```python
from build123d import *

# Parameters (mm, degrees)
SKETCH1_W           = 23
SKETCH1_H           = 12
BOSS_EXTRUDE1_DEPTH = 24
BOSS_EXTRUDE2_DEPTH = 4.5
SKETCH3_R           = 2.5
BOSS_EXTRUDE3_DEPTH = 3
SKETCH4_R           = 0.85
CUT_EXTRUDE1_DEPTH  = 5
BOSS_EXTRUDE4_START = -4
SKETCH5_W           = 4.5
SKETCH5_H           = 12
SKETCH5_R           = 1.125
BOSS_EXTRUDE4_DEPTH = 2.5


with BuildPart() as part:
    # Sketch1 → Boss-Extrude1 (new body)
    with BuildSketch(Plane(origin=(0, 0, 0), x_dir=(1, 0, 0), z_dir=(0, 1, 0))):
        Rectangle(SKETCH1_W, SKETCH1_H)
    extrude(amount=BOSS_EXTRUDE1_DEPTH)

    # Sketch2 → Boss-Extrude2 (add)
    with BuildSketch(Plane(origin=(0, 24, 0), x_dir=(1, 0, 0), z_dir=(0, 1, 0))):
        with BuildLine():
            ThreePointArc((0.303829175, 2.999968125), (-2.71, 0), (0.303829175, -2.999968125))
            ThreePointArc((0.303829175, -2.999968125), (11.5, 0), (0.303829175, 2.999968125))
        make_face()
    extrude(amount=BOSS_EXTRUDE2_DEPTH)

    # Sketch3 → Boss-Extrude3 (add)
    with BuildSketch(Plane(origin=(0, 28.5, 0), x_dir=(1, 0, 0), z_dir=(0, 1, 0))):
        with Locations(Location((5.5, 0, 0), (0, 0, 270))):
            Circle(SKETCH3_R)
    extrude(amount=BOSS_EXTRUDE3_DEPTH)

    # Sketch4 → Cut-Extrude1 (cut)
    with BuildSketch(Plane(origin=(0, 31.5, 0), x_dir=(1, 0, 0), z_dir=(0, 1, 0))):
        with Locations(Location((5.5, 0, 0), (0, 0, 270))):
            Circle(SKETCH4_R)
    extrude(amount=-CUT_EXTRUDE1_DEPTH, mode=Mode.SUBTRACT)

    # Sketch5 → Boss-Extrude4 (add)
    # profile 1 of 2: a face of its own
    with BuildSketch(Plane(origin=(0, 24, 0), x_dir=(1, 0, 0), z_dir=(0, 1, 0)).offset(BOSS_EXTRUDE4_START)):
        with Locations((-13.75, 0)):
            Rectangle(SKETCH5_W, SKETCH5_H)
        with Locations(Location((-13.75, 0, 0), (0, 0, 270))):
            Circle(SKETCH5_R, mode=Mode.SUBTRACT)
    # profile 2 of 2: a face of its own
    with BuildSketch(Plane(origin=(0, 24, 0), x_dir=(1, 0, 0), z_dir=(0, 1, 0)).offset(BOSS_EXTRUDE4_START)):
        with Locations((13.75, 0)):
            Rectangle(SKETCH5_W, SKETCH5_H)
        with Locations(Location((13.75, 0, 0), (0, 0, 90))):
            Circle(SKETCH5_R, mode=Mode.SUBTRACT)
    extrude(amount=-BOSS_EXTRUDE4_DEPTH)


solid = part.part
```
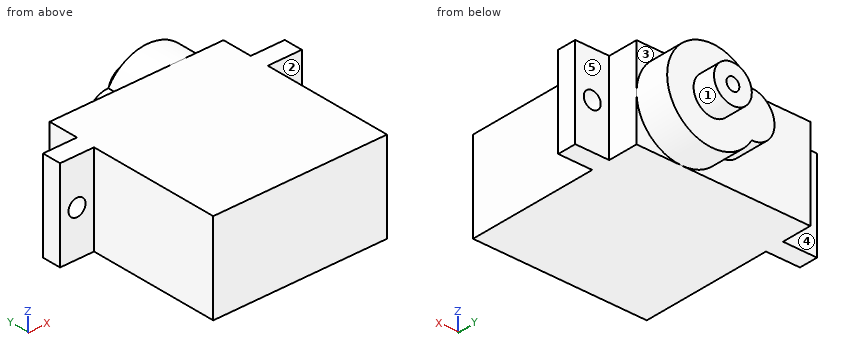
Part model, mm, in its own coordinate system. Face numbers are marked on the shaded views. A direction names the side the tool comes from. Coordinates: 2 decimals unless noted, no trailing zeros. Order: outer loops, then holes, each group sorted by start corner. A loop starts at its lowest first (then second) coordinate and runs counter-clockwise, first axis right, second up. Notation, with made-up numbers: (-8, 79.25) - (4, 79.25) arc R16 cw to (4, 87.25) - close; hole circle Ø3 at (84, 47). An arc over 180 degrees is marked (long way). Return JSON: item names as keys, results as strings. Group by question number.
Item 1: Cut at A-A (x = 13.75). List the corners of the cut face in (y, z) (3 decimals), plus the area to 3 significant figures.
Item 2: Pin check, flat tips, straight feed: pin 1 (5 mm diameter, centred on x = -6, z = -1, fed in from -Y); pin 2 (1.8 mm diameter, centred on x = 9.5, z = 2.5, fed in from +Y); pin 3 (0.8 mm diameter, centred on x = 5.5, z = 0, fed in from +Y); pin 4 (3.5 mm diameter, centred on x = -14, z = -2.5, fed in from +Y). Stop position of each tip, or through.
Item 3: Which spindle directions (+Z, -Z, +X, -X, +Y, -Y) get a long thin tool onto all of the face, cutting with end or side? Do the marked faces 1, 2, 3, 4 and 5. Say none if no direction does.
Item 4: Cut at D-D (y = 2.5). List the corners of the cut face in (x, z), plus the area to 3 significant figures.
Item 5: Cut at B-B (y = 18.5). List the corners of the cut face in (x, z) (3 decimals).
Item 6: Drill centre lines: probe 1 along X at (y, z) = (19.45, 0) (3 decimals); probe 2 along X at (y, z) = (8, 4.5); probe 3 along Y at (x, z) = (7.5, 5.75). Where is each one in solid material? Low to high. Write a range as from..to.
Item 7: Cut at C-C (z = -4). List the corners of the cut face in (x, y).
Check values:
{
 "1": {"outline": "(17.5, -6) - (20, -6) - (20, -1.125) - (17.5, -1.125) - close; (17.5, 1.125) - (20, 1.125) - (20, 6) - (17.5, 6) - close", "area": "24.4 mm2"},
 "2": {"pin 1": "stops at y = 0", "pin 2": "stops at y = 28.5", "pin 3": "stops at y = 26.5", "pin 4": "stops at y = 20"},
 "3": {"face 1": "+Y", "face 2": "+Z, -Z, +X, -Y", "face 3": "+Z, +X, +Y", "face 4": "+Z, -Z, -X, +Y", "face 5": "+Z, -Z, +X, +Y"},
 "4": {"outline": "(-11.5, -6) - (11.5, -6) - (11.5, 6) - (-11.5, 6) - close", "area": "276 mm2"},
 "5": {"outline": "(-16, -6) - (16, -6) - (16, 6) - (-16, 6) - close; hole circle Ø2.25 at (-13.75, 0); hole circle Ø2.25 at (13.75, 0)"},
 "6": {"probe 1": "x = -16..-14.875, -12.625..12.625, 14.875..16", "probe 2": "x = -11.5..11.5", "probe 3": "y = 0..24"},
 "7": {"outline": "(-16, 17.5) - (-11.5, 17.5) - (-11.5, 0) - (11.5, 0) - (11.5, 17.5) - (16, 17.5) - (16, 20) - (11.5, 20) - (11.5, 24) - (9.97, 24) - (9.97, 28.5) - (1.03, 28.5) - (1.03, 24) - (-11.5, 24) - (-11.5, 20) - (-16, 20) - close"}
}
